Geometry check sheet. Reference: the model listing, model coordinates, mm. A direction names the side the tool comes from. Round coordinates to 2 decimals unless told otherwise and drop trailing zeros. Loops run counter-clockwise (first coordinate to the right, second up) from the corner with the lowest first, then second, coordinate; pieces in that order, holes last. Notation, with made-up numbers: (83.25, 55) -> (128.25, 55) arc R14 cw to (128.25, 77) -> close; hole circle Ø9 at (18, 12). An arc over 180 degrees is marked (long way). Use a Markdown table: item, result. Add a question column.
Q1. Sectioned sample at B-B, the plane z = -8.5. Enter the section's corners in (x, y), then the cut area to 3 significant figures.
Q2. Sectioned sample at A-A, the plane z = 0. Enter the section's corners in (x, y), then the cut area to 4 significant figures.
Q3. Material ranges on L1, parallel to Y at x = 3, z = 0; L2, parallel to Z at x = -30.5, y = 9.5; L3, parallel to X at y = 0, z = 23.6, recorded low to high.
Q4. Release check for a two-part mould opening along Y. For faces 1 (the face through (-14.374, 1.318, 22.921)), 2 (the face through (6.35, 0, 0)), 3 (the face through (-24, -12.5, -22)) record: released by +Y, released by -Y, zero draft, split by the parting line, or undercut.
Q5. Sectioned sample at C-C, the plane x = -24. Enter the section's corners in (y, z), then the cut area to 4 significant figures.
Q6. Gauge pin test, flat ends, axial feed: P1, Ø4.5, axis at y = 0, z = -8.5, coming from the -X side; P2, Ø5, axis at x = -64.71, y = 0, coming from the +Z side; P3, Ø10, axis at y = 6, z = -19, coming from the -X side. Record the tip position at first contact, or that the pin passes through.
Q7. Set-up check for faces 4 (the face through (4.28, 0.59, 6.64)), 5 (the face through (-45.868, -3.178, -23.981)), 6 (the face through (-1.91, -0.18, 19.04)): record each of +Z, -Z, +X, -X, +Y, -Y from which the full face is reachable in a straight line by a thin tool's end or side.
Q8. Sectioned sample at D-D, the plane y = -8.5. Enter the section's corners in (x, z), then the cut area to 3 significant figures.
```python
from build123d import *

# Parameters (mm, degrees)
SKETCH2_W                                         = 29
SKETCH2_H                                         = 25
BOSS_EXTRUDE1_DEPTH                               = 6.35
CSK_FOR_M3_5_FLAT_HEAD_MACHINE_SCREW1_D           = 3.9
CSK_FOR_M3_5_FLAT_HEAD_MACHINE_SCREW1_CSINK_D     = 8.2
CSK_FOR_M3_5_FLAT_HEAD_MACHINE_SCREW1_CSINK_ANGLE = 90
EDGE_FLANGE1_DEPTH                                = 25
EDGE_FLANGE1_BEND_DEPTH                           = 25
CSK_FOR_M3_5_FLAT_HEAD_MACHINE_SCREW2_D           = 3.9
CSK_FOR_M3_5_FLAT_HEAD_MACHINE_SCREW2_DEPTH       = 6.35
CSK_FOR_M3_5_FLAT_HEAD_MACHINE_SCREW2_CSINK_D     = 8.2
CSK_FOR_M3_5_FLAT_HEAD_MACHINE_SCREW2_CSINK_ANGLE = 90
CUT_EXTRUDE1_DEPTH                                = 97.44393449
CUT_EXTRUDE2_DEPTH                                = 97.44393449


# Sheet-metal steps are written as plain solids
with BuildPart() as part:
    # Sketch2 → Boss-Extrude1 (new body)
    with BuildSketch(Plane(origin=(0, 0, 0), x_dir=(0, 0, -1), z_dir=(1, 0, 0))):
        Rectangle(SKETCH2_W, SKETCH2_H)
    extrude(amount=BOSS_EXTRUDE1_DEPTH)

    # CSK for M3.5 Flat Head Machine Screw1 (through all)
    with Locations(Plane.ZY):
        with Locations((0, -8.5), (8.5, 0), (0, 8.5), (-8.5, 0)):
            CounterSinkHole(CSK_FOR_M3_5_FLAT_HEAD_MACHINE_SCREW1_D / 2, CSK_FOR_M3_5_FLAT_HEAD_MACHINE_SCREW1_CSINK_D / 2, counter_sink_angle=CSK_FOR_M3_5_FLAT_HEAD_MACHINE_SCREW1_CSINK_ANGLE)

    # Edge-Flange1 section (across the edge) → Edge-Flange1 (add)
    with BuildSketch(Plane(origin=(0, 12.5, -20.85), x_dir=(0, 0, 1), z_dir=(0, -1, 0))):
        with BuildLine():
            Line((-6.35, 6.35), (-6.35, 78.65))
            Line((-6.35, 78.65), (0, 78.65))
            Line((0, 78.65), (0, 6.35))
            ThreePointArc((0, 6.35), (1.859871939, 1.859871939), (6.35, 0))
            Line((6.35, 0), (6.35, -6.35))
            ThreePointArc((6.35, -6.35), (-2.630256121, -2.630256121), (-6.35, 6.35))
        make_face()
    extrude(amount=EDGE_FLANGE1_DEPTH)

    # Edge-Flange1 section 2 (across the edge) → Edge-Flange1 bend (add)
    with BuildSketch(Plane(origin=(0, -12.5, 20.85), x_dir=(0, 0, -1), z_dir=(0, 1, 0))):
        with BuildLine():
            Line((-6.35, 6.35), (-6.35, 78.65))
            Line((-6.35, 78.65), (0, 78.65))
            Line((0, 78.65), (0, 6.35))
            ThreePointArc((0, 6.35), (1.859871939, 1.859871939), (6.35, 0))
            Line((6.35, 0), (6.35, -6.35))
            ThreePointArc((6.35, -6.35), (-2.630256121, -2.630256121), (-6.35, 6.35))
        make_face()
    extrude(amount=EDGE_FLANGE1_BEND_DEPTH)

    # CSK for M3.5 Flat Head Machine Screw2
    with Locations(Plane.XY.offset(27.2)):
        with Locations((-64.709225, 0), (-15.810775, 0)):
            csk_for_m3_5_flat_head_machine_screw2 = CounterSinkHole(CSK_FOR_M3_5_FLAT_HEAD_MACHINE_SCREW2_D / 2, CSK_FOR_M3_5_FLAT_HEAD_MACHINE_SCREW2_CSINK_D / 2, depth=CSK_FOR_M3_5_FLAT_HEAD_MACHINE_SCREW2_DEPTH, counter_sink_angle=CSK_FOR_M3_5_FLAT_HEAD_MACHINE_SCREW2_CSINK_ANGLE)

    # Mirror1: CSK for M3.5 Flat Head Machine Screw2 across plane
    add(csk_for_m3_5_flat_head_machine_screw2.mirror(Plane.XY), mode=Mode.SUBTRACT)

    # Sketch20 → Cut-Extrude1 (cut, through all)
    with BuildSketch(Plane.XY.offset(27.2)):
        Polygon((-32.817666355, 0), (-36.538833178, 6.44525), (-43.981166822, 6.44525), (-47.702333645, 0), (-43.981166822, -6.44525), (-36.538833178, -6.44525), align=None)
    extrude(amount=-CUT_EXTRUDE1_DEPTH, mode=Mode.SUBTRACT)

    # Sketch21 → Cut-Extrude2 (cut, through all)
    with BuildSketch(Plane.XY.offset(27.2)):
        with BuildLine():
            Line((-64.709225, -12.5), (-78.65, -12.5))
            Line((-78.65, -12.5), (-78.65, 12.5))
            Line((-78.65, 12.5), (-64.709225, 12.5))
            ThreePointArc((-64.709225, 12.5), (-77.209225, 0), (-64.709225, -12.5))
        make_face()
    extrude(amount=-CUT_EXTRUDE2_DEPTH, mode=Mode.SUBTRACT)


solid = part.part
```
Values:
| question | item | result |
|---|---|---|
| 1 | outline | (0, -12.5) -> (6.35, -12.5) -> (6.35, -1.95) -> (2.15, -1.95) -> (0, -4.1) -> close; (0, 4.1) -> (2.15, 1.95) -> (6.35, 1.95) -> (6.35, 12.5) -> (0, 12.5) -> close |
| 1 | area | 129 mm^2 |
| 2 | outline | (0, -4.4) -> (2.15, -6.55) -> (6.35, -6.55) -> (6.35, 6.55) -> (2.15, 6.55) -> (0, 4.4) -> close; (0.1, -12.5) -> (6.35, -12.5) -> (6.35, -10.45) -> (2.15, -10.45) -> close; (0.1, 12.5) -> (2.15, 10.45) -> (6.35, 10.45) -> (6.35, 12.5) -> close |
| 2 | area | 100.0 mm^2 |
| 3 | L1 | -12.5 to -10.45, -6.55 to 6.55, 10.45 to 12.5 |
| 3 | L2 | -27.2 to -20.85, 20.85 to 27.2 |
| 3 | L3 | -77.21 to -66.66, -62.76 to -47.7, -32.82 to -17.76, -13.86 to 2.51 |
| 4 | face 1 | undercut |
| 4 | face 2 | zero draft |
| 4 | face 3 | released by -Y |
| 5 | outline | (-12.5, -27.2) -> (12.5, -27.2) -> (12.5, -20.85) -> (-12.5, -20.85) -> close; (-12.5, 20.85) -> (12.5, 20.85) -> (12.5, 27.2) -> (-12.5, 27.2) -> close |
| 5 | area | 317.5 mm^2 |
| 6 | P1 | x = 1.85 |
| 6 | P2 | z = 25.6 |
| 6 | P3 | x = -77.14 |
| 7 | face 4 | +X, -X |
| 7 | face 5 | +Z, -Z |
| 7 | face 6 | -X, +Y, -Y |
| 8 | outline | (-73.87, -27.2) -> (-6.35, -27.2) arc R12.7 ccw to (6.35, -14.5) -> (6.35, -1.95) -> (2.15, -1.95) -> (0, -4.1) -> (0, -14.5) arc R6.35 cw to (-6.35, -20.85) -> (-73.87, -20.85) -> close; (-73.87, 20.85) -> (-6.35, 20.85) arc R6.35 cw to (0, 14.5) -> (0, 4.1) -> (2.15, 1.95) -> (6.35, 1.95) -> (6.35, 14.5) arc R12.7 ccw to (-6.35, 27.2) -> (-73.87, 27.2) -> close |
| 8 | area | 1,200 mm^2 |
